from build123d import *

# Parameters (mm, degrees)
EXTRUDE_1_DEPTH          = 8
EXTRUDE_START            = 4
EXTRUDE_2_DEPTH          = 4
EXTRUDE_3_DEPTH          = 22
CUT_EXTRUDE_1_DEPTH      = 65.412731661
CUT_EXTRUDE_1_DEPTH_BACK = 65.412731661


with BuildPart() as part:
    # Sketch 1 → Extrude 1 (new body)
    # profile 1 of 3: a face of its own
    with BuildSketch(Plane.XY):
        with BuildLine():
            Line((-27.592823234, 10), (-27.592823234, 2))
            Line((-27.592823234, 2), (4.407176766, 2))
            Line((4.407176766, 2), (4.407176766, 11))
            ThreePointArc((4.407176766, 11), (6.753152543, 18.127398986), (12.873812817, 22.468013743))
            Line((12.873812817, 22.468013743), (-27.592823234, 10))
        make_face()
    # profile 2 of 3: a face of its own
    with BuildSketch(Plane.XY):
        Polygon((-27.592823234, -10), (28.407176766, -10), (28.407176766, -2), (4.407176766, -2), (4.407176766, 2), (-27.592823234, 2), align=None)
    # profile 3 of 3: a face of its own
    with BuildSketch(Plane.XY):
        with BuildLine():
            Line((4.407176766, -2), (28.407176766, -2))
            Line((28.407176766, -2), (28.407176766, 11))
            ThreePointArc((28.407176766, 11), (23.534575752, 20.654024223), (12.873812817, 22.468013743))
            ThreePointArc((12.873812817, 22.468013743), (6.753152543, 18.127398986), (4.407176766, 11))
            Line((4.407176766, 11), (4.407176766, 2))
            Line((4.407176766, 2), (4.407176766, -2))
        make_face()
        with BuildLine():
            ThreePointArc((10.407176766, 11), (16.407176766, 17), (22.407176766, 11))
            Line((22.407176766, 11), (22.407176766, 6))
            ThreePointArc((22.407176766, 6), (16.407176766, 0), (10.407176766, 6))
            Line((10.407176766, 6), (10.407176766, 11))
        make_face(mode=Mode.SUBTRACT)
    extrude(amount=-EXTRUDE_1_DEPTH)

    # Sketch 1_3 → Extrude 2 (add)
    with BuildSketch(Plane.XY.offset(EXTRUDE_START)):
        with BuildLine():
            Line((4.407176766, -2), (28.407176766, -2))
            Line((28.407176766, -2), (28.407176766, 11))
            ThreePointArc((28.407176766, 11), (23.534575752, 20.654024223), (12.873812817, 22.468013743))
            ThreePointArc((12.873812817, 22.468013743), (6.753152543, 18.127398986), (4.407176766, 11))
            Line((4.407176766, 11), (4.407176766, 2))
            Line((4.407176766, 2), (4.407176766, -2))
        make_face()
        with BuildLine():
            ThreePointArc((10.407176766, 11), (16.407176766, 17), (22.407176766, 11))
            Line((22.407176766, 11), (22.407176766, 6))
            ThreePointArc((22.407176766, 6), (16.407176766, 0), (10.407176766, 6))
            Line((10.407176766, 6), (10.407176766, 11))
        make_face(mode=Mode.SUBTRACT)
    extrude(amount=-EXTRUDE_2_DEPTH)

    # Sketch 1_4 → Extrude 3 (add)
    with BuildSketch(Plane.XY):
        Polygon((-27.592823234, -10), (28.407176766, -10), (28.407176766, -2), (4.407176766, -2), (4.407176766, 2), (-27.592823234, 2), align=None)
    extrude(amount=EXTRUDE_3_DEPTH)

    # Sketch 3 → Cut-Extrude 1 (cut, two sides: drawn at the far end of the back side and taken through both)
    with BuildSketch(Plane.ZY.offset(27.592823234).offset(-CUT_EXTRUDE_1_DEPTH_BACK)):
        Polygon((2, -10), (-0.886751346, -5), (14.886751346, -5), (12, -10), align=None)
    extrude(amount=CUT_EXTRUDE_1_DEPTH + CUT_EXTRUDE_1_DEPTH_BACK, mode=Mode.SUBTRACT)


solid = part.part
For this review, take the finished solid that the model builds, in its own axes (mm). A direction names the side the tool comes from. Round coordinates to 2 decimals unless told otherwise and drop trailing zeros. Loops run counter-clockwise (first coordinate to the right, second up) from the corner with the lowest first, then second, coordinate; pieces in that order, holes last. Notation, with made-up numbers: (16.5, 75) - (25.5, 75) arc R20 cw to (25.5, 83) - close; hole circle Ø5 at (35, 79.5). An arc over 180 degrees is marked (long way). Use one line per item in the form item = value.
Item 1: Consider section D-D on y = -6.5. Write out the cut boundary in (x, z), then the cut area to 3 significant figures.
Answers:
outline = (-27.59, -8) - (28.41, -8) - (28.41, -0.02) - (-27.59, -0.02) - close; (-27.59, 14.02) - (28.41, 14.02) - (28.41, 22) - (-27.59, 22) - close
area = 894 mm^2
Item 2: Consider section A-A on y = 13.5. Write out the cut boundary in (x, z), then the cut area to 3 significant figures.
Answers:
outline = (-16.23, -8) - (10.95, -8) - (10.95, 4) - (4.67, 4) - (4.67, 0) - (-16.23, 0) - close; (21.86, -8) - (28.14, -8) - (28.14, 4) - (21.86, 4) - close
area = 318 mm^2
Item 3: Tool access review of faces 5 (the flat face through (-8, 10, 0)), 6 (the flat face through (4.407, 0, 13)), 7 (the flat face through (22.407, 9, -2)): name each direction out of +Z, -Z, +X, -X, +Y, -Y from which nothing blocks a thin tool from reaching the whole face with its end or side.
Answers:
face_5 = +Z, -X, +Y
face_6 = +Z, +X, +Y
face_7 = +Z, -Z
Item 4: Consider section B-B on x = -19. Write out the cut boundary in (y, z), then the cut area to 3 significant figures.
Answers:
outline = (-10, -8) - (12.65, -8) - (12.65, 0) - (2, 0) - (2, 22) - (-10, 22) - (-10, 12) - (-5, 14.89) - (-5, -0.89) - (-10, 2) - close
area = 381 mm^2
Item 5: For line 1 (Y direction, x = 17, z = 1.25); line 2 (Y direction, x = 17.5, z = 7.25); line 3 (Y direction, x = -22, z = 18.75), list the stretches that pass through material, from the lowest coordinate up.
Answers:
line_1 = -10 to -8.7, -5 to 0.03, 16.97 to 22.99
line_2 = -5 to -2
line_3 = -10 to 2
Item 6: Mouldability with a two-part tool opening along X and no side actions: class faces 1 (the flat face through (-11, 2, 11)), 2 (the flat face through (28.407, 0, 3)), 3 (the cylindrical face through (16.3, 17, -1.9)), 4 (the flat face through (4.407, 7, 2)) as +X half, -X half, draft (parallel to the pull), parting line (faces both ways), or undercut.
Answers:
face_1 = draft
face_2 = +X half
face_3 = undercut
face_4 = -X half
Item 7: Consider section C-C on z = 7.5. Write out the cut boundary in (x, y).
Answers:
outline = (-27.59, -5) - (28.41, -5) - (28.41, -2) - (4.41, -2) - (4.41, 2) - (-27.59, 2) - close
Item 8: Clearance check with flat-ended pins moving along their axes: P1, Ø1, axis at x = 6, y = 9.5, coming from the +Z side; P2, Ø3, axis at y = 17, z = 2, coming from the -X side; P3, Ø2, axis at y = 5.5, z = 2.5, coming from the -X side. State where each tip first meets the part, or that it passes through.
Answers:
P1 = 4
P2 = 5.28
P3 = 4.41
